from build123d import *

# Parameters (mm, degrees)
SKETCH1_W           = 20
SKETCH1_H           = 20
BOSS_EXTRUDE1_DEPTH = 20
SKETCH2_R           = 7.5
CUT_EXTRUDE1_DEPTH  = 20
SKETCH3_R           = 7.5
SKETCH3_R_2         = 6.5
BOSS_EXTRUDE2_DEPTH = 3


with BuildPart() as part:
    # Sketch1 → Boss-Extrude1 (new body)
    with BuildSketch(Plane.XY):
        with Locations((10, 10)):
            Rectangle(SKETCH1_W, SKETCH1_H)
    extrude(amount=BOSS_EXTRUDE1_DEPTH)

    # Sketch2 → Cut-Extrude1 (cut)
    with BuildSketch(Plane(origin=(20, 0, 0), x_dir=(0, 0, -1), z_dir=(1, 0, 0))):
        with Locations((-10, 10)):
            Circle(SKETCH2_R)
    extrude(amount=-CUT_EXTRUDE1_DEPTH, mode=Mode.SUBTRACT)

    # Sketch3 → Boss-Extrude2 (add)
    with BuildSketch(Plane(origin=(0, 0, 0), x_dir=(-1, 0, 0), z_dir=(0, -1, 0))):
        with Locations(Location((-10, -10, 0), (0, 0, 270))):
            Circle(SKETCH3_R)
        with Locations(Location((-10, -10, 0), (0, 0, 90))):
            Circle(SKETCH3_R_2, mode=Mode.SUBTRACT)
    extrude(amount=BOSS_EXTRUDE2_DEPTH)


solid = part.part
The listing builds one solid part. Answer for the finished solid, in the listing's coordinates (mm). A direction names the side the tool comes from. Give positions to 0.01 mm unless a question says otherwise; leave off trailing zeros. Write each loop counter-clockwise with the first axis right and the second up, starting at its lowest first coordinate (ties: lowest second). Pieces come first, ordered by that corner, then holes. Notation, with made-up numbers: (22, -10) - (27, -10) arc R27 cw to (27, 28) - close; hole circle Ø10 at (61, 57.5). An arc over 180 degrees is marked (long way). One line per question, with ' | ' between items. Start each with the question number.
1. Section D-D, the plane y = 7.5 is taken. Determine the outline of the cut face in (x, z).
2. Straight lines are drawn through the part: line 1 (X direction, y = -2.15, z = 10); line 2 (Y direction, x = 12, z = 2); line 3 (Y direction, x = 12.75, z = 10). For each, find the intervals that lie inside material, in ascending order.
3. Given P1, Ø6.5, axis at x = 7.5, z = 11.5, coming from the -Y side, flat-ended and moving along its own axis, determine where the tip first touches the part or whether it passes through.
4. Section B-B, the plane y = 10 is taken. Determine the outline of the cut face in (x, z).
5. Determine the mould class of faces 3 (the face through (10, 20, 10)), 4 (the face through (11.95, -1.48, 3.8)), 5 (the face through (9.67, -1.479, 2.507)) for opening direction X: +X half, -X half, draft (parallel to the pull), parting line (faces both ways), or undercut.
6. Section A-A, the plane z = 10 is taken. Determine the outline of the cut face in (x, y).
7. Section C-C, the plane x = 10 is taken. Determine the outline of the cut face in (y, z).
8. For faces 1 (the face through (10, 0, 10)), 2 (the face through (0, 5, 3)), determine the directions among +Z, -Z, +X, -X, +Y, -Y from which every point of the face is accessible in a straight line to the end or side of a thin tool.
Result:
1) outline: (0, 0) - (20, 0) - (20, 2.93) - (0, 2.93) - close; (0, 17.07) - (20, 17.07) - (20, 20) - (0, 20) - close
2) line 1: x = 2.5 to 3.5, 16.5 to 17.5 | line 2: y = 0 to 20 | line 3: y = 0 to 2.5, 17.5 to 20
3) P1: stops at y = 0
4) outline: (0, 0) - (20, 0) - (20, 2.5) - (0, 2.5) - close; (0, 17.5) - (20, 17.5) - (20, 20) - (0, 20) - close
5) face 3: draft | face 4: undercut | face 5: parting line
6) outline: (0, 0) - (2.5, 0) - (2.5, -3) - (3.5, -3) - (3.5, 0) - (16.5, 0) - (16.5, -3) - (17.5, -3) - (17.5, 0) - (20, 0) - (20, 2.5) - (0, 2.5) - close; (0, 17.5) - (20, 17.5) - (20, 20) - (0, 20) - close
7) outline: (-3, 2.5) - (0, 2.5) - (0, 0) - (20, 0) - (20, 20) - (0, 20) - (0, 17.5) - (-3, 17.5) - (-3, 16.5) - (0, 16.5) - (0, 3.5) - (-3, 3.5) - close; hole circle Ø15 at (10, 10)
8) face 1: -Y | face 2: +Z, -Z, -X, +Y, -Y
